from build123d import *

# Parameters (mm, degrees)
SKETCH1_W               = 15
SKETCH1_H               = 4
FILLET3_R               = 2
CUT_EXTRUDE1_DEPTH      = 81.833161512
CUT_EXTRUDE1_DEPTH_BACK = 81.833161512
SKETCH2_R               = 1.25


with BuildPart() as part:
    # Sketch1 → Revolve2 (revolve)
    with BuildSketch(Plane.XY):
        with Locations((7.5, 76)):
            Rectangle(SKETCH1_W, SKETCH1_H)
        Polygon((0, 74), (0, 0), (10.049031003, 0), (10.049031003, 64), (15, 64), (15, 74), align=None)
    revolve(axis=Axis((0, 0, 0), (0, 1, 0)))

    # Fillet3
    fillet3_edges = [part.edges().sort_by_distance(p)[0] for p in [
        (-15, 78, 0),
    ]]
    fillet(fillet3_edges, radius=FILLET3_R)

    # Sketch2 → Cut-Extrude1 (cut, two sides: drawn at the far end of the back side and taken through both)
    with BuildSketch(Plane.XY.offset(-CUT_EXTRUDE1_DEPTH_BACK)):
        with Locations(Location((0.049031003, 7, 0), (0, 0, 180))):
            Circle(SKETCH2_R)
    extrude(amount=CUT_EXTRUDE1_DEPTH + CUT_EXTRUDE1_DEPTH_BACK, mode=Mode.SUBTRACT)


solid = part.part
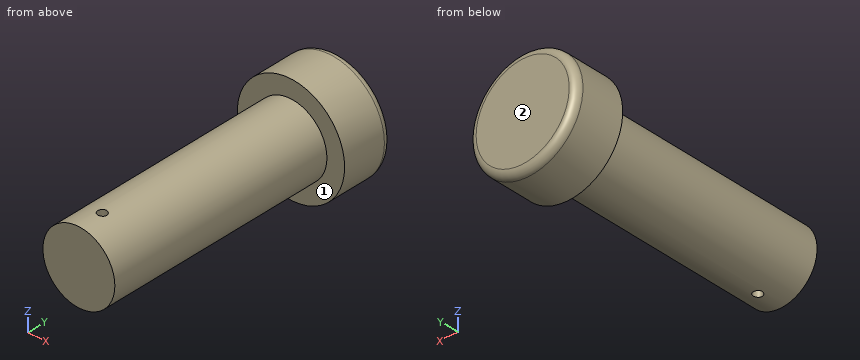
The listing builds one solid part. Answer for the finished solid, in the listing's coordinates (mm). Face numbers are marked on the shaded views. A direction names the side the tool comes from. Coordinates: 2 decimals unless noted, no trailing zeros. Loops run counter-clockwise (first coordinate to the right, second up) from the corner with the lowest first, then second, coordinate; pieces in that order, holes last.
1) Find section D-D on y = 37.5. Write down the section's boundary in (x, z), then the cut area to 3 significant figures.
2) Find the intervals of material crossed by L1, parallel to Y at x = 0, z = 7.75; L2, parallel to Z at x = 0.25, y = 4; L3, parallel to Y at x = -0.25, z = -10.25, in increasing order.
3) Find section C-C on y = 7. Write down the section's boundary in (x, z).
4) Find section B-B on z = 0. Write down the section's boundary in (x, y).
5) A tool of negligible diameter and unlimited length cuts with its end or side. For the marked faces 1 and 2, from which of +Z, -Z, +X, -X, +Y, -Y can it reach the whole face along a straight path? Write none if from no direction.
6) Flat-ended cylindrical pins translate along their axes: pin 1 Ø1.5 at (y, z) = (21, 7.5) entering from +X; pin 2 Ø4 at (x, y) = (5, 62.5) entering from -Z; pin 3 Ø1 at (y, z) = (56, -4) entering from +X. Find the tip coordinate at first contact, or state that the pin passes through.
7) Find section A-A on x = 0. Write down the section's boundary in (y, z).
Values:
1. outline: circle Ø20.1 at (0, 0)
1. area: 317 mm2
2. L1: y = 0 to 5.75, 8.25 to 78
2. L2: z = -10.05 to 10.05
2. L3: y = 64 to 78
3. outline: (-1.2, -9.98) - (-1.2, 9.98) arc R10.05 ccw to start; (1.3, -9.96) arc R10.05 ccw to (1.3, 9.96) - close
4. outline: (-15, 64) - (-10.05, 64) - (-10.05, 0) - (10.05, 0) - (10.05, 64) - (15, 64) - (15, 76) arc R2 ccw to (13, 78) - (-13, 78) arc R2 ccw to (-15, 76) - close; hole circle Ø2.5 at (0.05, 7)
5. face 1: -Y
5. face 2: +Z, -Z, +X, -X, +Y
6. pin 1: stops at x = 7.44
6. pin 2: stops at z = -14.54
6. pin 3: stops at x = 9.42
7. outline: (0, -10.05) - (5.75, -10.05) - (5.75, 10.05) - (0, 10.05) - close; (8.25, -10.05) - (64, -10.05) - (64, -15) - (76, -15) arc R2 ccw to (78, -13) - (78, 13) arc R2 ccw to (76, 15) - (64, 15) - (64, 10.05) - (8.25, 10.05) - close
